```python
from build123d import *

# Parameters (mm, degrees)
SKETCH1_W               = 40
SKETCH1_H               = 140
BOSS_EXTRUDE1_DEPTH     = 8
SKETCH2_W               = 10.491495072
SKETCH2_H               = 43.818703547
SKETCH2_W_2             = 11.094869632
SKETCH2_H_2             = 36.296784829
CUT_EXTRUDE1_DEPTH      = 1
CUT_EXTRUDE1_DEPTH_BACK = 9
FILLET3_R               = 8
FILLET4_R               = 4
SKETCH3_R               = 1.5
CUT_EXTRUDE2_DEPTH      = 1
CUT_EXTRUDE2_DEPTH_BACK = 9
SKETCH4_W               = 15.7
SKETCH4_H               = 0.9
CUT_EXTRUDE3_DEPTH      = 12.094869632
CUT_EXTRUDE3_DEPTH_BACK = 29.905130368
SKETCH5_R               = 3.05
CUT_EXTRUDE4_DEPTH      = 5.5
SKETCH6_R               = 2
CUT_EXTRUDE5_DEPTH      = 1
CUT_EXTRUDE5_DEPTH_BACK = 9
SKETCH7_R               = 5
CUT_EXTRUDE6_DEPTH      = 3.5


with BuildPart() as part:
    # Sketch1 → Boss-Extrude1 (new body)
    with BuildSketch(Plane(origin=(0, 0, 0), x_dir=(1, 0, 0), z_dir=(0, 1, 0))):
        Rectangle(SKETCH1_W, SKETCH1_H)
    extrude(amount=BOSS_EXTRUDE1_DEPTH)

    # Sketch2 → Cut-Extrude1 (cut, two sides)
    with BuildSketch(Plane(origin=(0, 8, 0), x_dir=(1, 0, 0), z_dir=(0, 1, 0))) as cut_extrude1_sk:
        with Locations((14.754252464, 48.090648227)):
            Rectangle(SKETCH2_W, SKETCH2_H)
        with Locations((-14.452565184, -51.851607586)):
            Rectangle(SKETCH2_W_2, SKETCH2_H_2)
        with Locations((14.452565184, -51.851607586)):
            Rectangle(SKETCH2_W_2, SKETCH2_H_2)
        with Locations((-14.754252464, 48.090648227)):
            Rectangle(SKETCH2_W, SKETCH2_H)
    extrude(amount=CUT_EXTRUDE1_DEPTH, mode=Mode.SUBTRACT)
    extrude(cut_extrude1_sk.sketch, amount=-CUT_EXTRUDE1_DEPTH_BACK, mode=Mode.SUBTRACT)

    # Fillet3
    fillet3_edges = [part.edges().sort_by_distance(p)[0] for p in [
        (-9.508504928, 4, -70),
        (8.905130368, 4, 70),
        (-8.905130368, 4, 70),
        (9.508504928, 4, -70),
    ]]
    fillet(fillet3_edges, radius=FILLET3_R)

    # Fillet4
    fillet4_edges = [part.edges().sort_by_distance(p)[0] for p in [
        (-9.508504928, 4, -26.181296453),
        (-20, 4, -26.181296453),
        (8.905130368, 4, 33.703215171),
        (20, 4, 33.703215171),
        (-8.905130368, 4, 33.703215171),
        (-20, 4, 33.703215171),
        (9.508504928, 4, -26.181296453),
        (20, 4, -26.181296453),
    ]]
    fillet(fillet4_edges, radius=FILLET4_R)

    # Sketch3 → Cut-Extrude2 (cut, two sides)
    with BuildSketch(Plane(origin=(0, 8, 0), x_dir=(1, 0, 0), z_dir=(0, 1, 0))) as cut_extrude2_sk:
        with Locations((12.5, -6.862591123)):
            Circle(SKETCH3_R)
        with Locations((0, 5.637408877)):
            Circle(SKETCH3_R)
        with Locations((-12.5, -6.862591123)):
            Circle(SKETCH3_R)
        with Locations((0, -19.362591123)):
            Circle(SKETCH3_R)
    extrude(amount=CUT_EXTRUDE2_DEPTH, mode=Mode.SUBTRACT)
    extrude(cut_extrude2_sk.sketch, amount=-CUT_EXTRUDE2_DEPTH_BACK, mode=Mode.SUBTRACT)

    # Sketch4 → Cut-Extrude3 (cut, two sides)
    with BuildSketch(Plane(origin=(8.905130368, 0, 0), x_dir=(0, 0, -1), z_dir=(1, 0, 0))) as cut_extrude3_sk:
        with Locations((-44.089134708, 0.45)):
            Rectangle(SKETCH4_W, SKETCH4_H)
    extrude(amount=CUT_EXTRUDE3_DEPTH, mode=Mode.SUBTRACT)
    extrude(cut_extrude3_sk.sketch, amount=-CUT_EXTRUDE3_DEPTH_BACK, mode=Mode.SUBTRACT)

    # Sketch5 → Cut-Extrude4 (cut)
    with BuildSketch(Plane.XZ):
        with Locations((12.5, 6.862591123)):
            Circle(SKETCH5_R)
        with Locations((0, -5.637408877)):
            Circle(SKETCH5_R)
        with Locations((-12.5, 6.862591123)):
            Circle(SKETCH5_R)
        with Locations((0, 19.362591123)):
            Circle(SKETCH5_R)
    extrude(amount=-CUT_EXTRUDE4_DEPTH, mode=Mode.SUBTRACT)

    # Sketch6 → Cut-Extrude5 (cut, two sides)
    with BuildSketch(Plane.XZ) as cut_extrude5_sk:
        with Locations((0, 60)):
            Circle(SKETCH6_R)
        with Locations((0, -55)):
            Circle(SKETCH6_R)
        with Locations((0, -40)):
            Circle(SKETCH6_R)
    extrude(amount=CUT_EXTRUDE5_DEPTH, mode=Mode.SUBTRACT)
    extrude(cut_extrude5_sk.sketch, amount=-CUT_EXTRUDE5_DEPTH_BACK, mode=Mode.SUBTRACT)

    # Sketch7 → Cut-Extrude6 (cut)
    with BuildSketch(Plane(origin=(0, 8, 0), x_dir=(1, 0, 0), z_dir=(0, 1, 0))):
        with Locations((0, 55)):
            Circle(SKETCH7_R)
        with Locations((0, -60)):
            Circle(SKETCH7_R)
        with Locations((0, 40)):
            Circle(SKETCH7_R)
    extrude(amount=-CUT_EXTRUDE6_DEPTH, mode=Mode.SUBTRACT)


solid = part.part
```
The listing builds one solid part. Answer for the finished solid, in the listing's coordinates (mm). A direction names the side the tool comes from. Coordinates: 2 decimals unless noted, no trailing zeros. Write each loop counter-clockwise with the first axis right and the second up, starting at its lowest first coordinate (ties: lowest second). Pieces come first, ordered by that corner, then holes.
Q1. Find the intervals of material crossed by line 1 along Z through (x, y) = (0, 1.5); line 2 along X through (y, z) = (3.5, 6.5); line 3 along X through (y, z) = (0.5, -53.5), in increasing order.
Returned:
line 1: z = -70 to -57, -53 to -42, -38 to -8.69, -2.59 to 16.31, 22.41 to 58, 62 to 70
line 2: x = -20 to -15.53, -9.47 to 9.47, 15.53 to 20
line 3: x = -9.51 to -1.32, 1.32 to 9.51
Q2. Which of the six approach directions +Z, -Z, +X, -X, +Y, -Y give full straight-line access (tool end or side, diameter ignored) to faces 4 (the cylindrical face through (-0.651, 6.274, -59.957)), 5 (the flat face through (9.509, 4, -46)), 6 (the cylindrical face through (-14.75, 2.71, 8.92))?
Returned:
face 4: +Y
face 5: -Z, +X, +Y, -Y
face 6: -Y
Q3. Section A-A, the plane z = -40 is taken. Write down the section's boundary in (x, y), then the cut area to 3 significant figures.
Returned:
outline: (-9.51, 0) - (-2, 0) - (-2, 4.5) - (-5, 4.5) - (-5, 8) - (-9.51, 8) - close; (2, 0) - (9.51, 0) - (9.51, 8) - (5, 8) - (5, 4.5) - (2, 4.5) - close
area: 99.1 mm2
Q4. Section B-B, the plane y = 2.5 is taken. Give the number of separate pieces and of enclosed holes in the cut face, then the cut area to 3 significant figures.
Returned:
separate pieces: 1
enclosed holes: 7
area: 3,670 mm2
Q5. Section C-C, the plane z = 40.5 is taken. Write down the section's boundary in (x, y), then the cut area to 3 significant figures.
Returned:
outline: (-8.91, 0.9) - (8.91, 0.9) - (8.91, 8) - (-8.91, 8) - close
area: 126 mm2
Q6. Section D-D, the plane z = 60 is taken. Write down the section's boundary in (x, y).
Returned:
outline: (-8.91, 0) - (-2, 0) - (-2, 4.5) - (-5, 4.5) - (-5, 8) - (-8.91, 8) - close; (2, 0) - (8.91, 0) - (8.91, 8) - (5, 8) - (5, 4.5) - (2, 4.5) - close
Q7. Given P1, Ø4.5, axis at x = -0.5, z = 42.5, coming from the -Y side; P2, Ø3, axis at x = -0.5, z = -6.5, coming from the -Y side; P3, Ø1.5, axis at x = 14.5, y = 3.5, coming from the +Z side, each flat-ended and moving along its own axis, determine where each tip first touches the part or whether it passes through.
Returned:
P1: stops at y = 0.9
P2: stops at y = 5.5
P3: stops at z = 33.7
Q8. The mould has two halves that part along Z. Classify faces 1 (the flat face through (4, 0, -6)), 2 (the flat face through (0, 0.9, 44)), 3 (the cylindrical face through (-18.8, 3.94, -25.04)): released by +Z, released by -Z, zero draft, split by the parting line, or undercut.
Returned:
face 1: zero draft
face 2: undercut
face 3: released by -Z
